```python
from build123d import *

# Parameters (mm, degrees)
F0_W      = 30
F0_H      = 30
F1_DEPTH  = 7
F3_DEPTH  = 7
F3_FACE_W = 4
F3_FACE_H = 7
F4_DEPTH  = 8


with BuildPart() as f1:
    # F0 (on Top) → F1 (new body)
    with BuildSketch(Plane.XY):
        Rectangle(F0_W, F0_H)
    extrude(amount=F1_DEPTH)

    # F2 (on face) → F3 (join)
    with BuildSketch(Plane.XY.offset(7)):
        with BuildLine():
            ThreePointArc((4, 0), (0, -4), (-4, 0))
            Line((-4, 0), (-8, 0))
            ThreePointArc((-8, 0), (0, -8), (8, 0))
            Line((8, 0), (4, 0))
        make_face()
    extrude(amount=F3_DEPTH)

    # F3_face (on face) → F4 (join)
    with BuildSketch(Plane(origin=(-6, 0, 10.5), x_dir=(-1, 0, 0), z_dir=(0, 1, 0))):
        Rectangle(F3_FACE_W, F3_FACE_H)
        with Locations((-12, 0)):
            Rectangle(F3_FACE_W, F3_FACE_H)
    extrude(amount=F4_DEPTH)


solid = f1.part
```
Work out the finished part from the listing and answer in its coordinate system (mm). A direction names the side the tool comes from. Give positions to 0.01 mm unless a question says otherwise; leave off trailing zeros. Loops run counter-clockwise (first coordinate to the right, second up) from the corner with the lowest first, then second, coordinate; pieces in that order, holes last. Notation, with made-up numbers: M -6.75,-6 L 39.25,-6 A15 cw 39.25,-1 Z; hole C -13,44.5 d2. An arc over 180 degrees is marked long. One line per item, written item: value. Start each with the question number.
1. Find section A-A (x = 0). Give the vertices of the cut face in (y, z).
2. Find section C-C (z = 11.5). Give the vertices of the cut face in (x, y), and give its area (3 significant figures).
3. Find section D-D (x = -9). Give the vertices of the cut face in (y, z), and give its area (3 significant figures).
4. Find section B-B (y = 7). Give the vertices of the cut face in (x, z).
5. Determine the mould class of faces 5 (the face through (-15, 0, 3)), 6 (the face through (0, 0, 0)), 7 (the face through (15, 0, 3)), 8 (the face through (0, 0, 7)) for opening direction X: released by +X, released by -X, zero draft, split by the parting line, or undercut.
6. Find the intervals of material crossed by probe 1 along X at (y, z) = (3, 12); probe 2 along Z at (x, y) = (3.5, 1); probe 3 along Y at (x, z) = (0, 9.25), in increasing order.
7. Which of the six approach directions +Z, -Z, +X, -X, +Y, -Y give full straight-line access (tool end or side, diameter ignored) to faces 1 (the face through (0, -8, 10)), 2 (the face through (-8, 4, 10)), 3 (the face through (4, 4, 10)), 4 (the face through (6, 8, 11))?
8. Each of these flat-tipped pins is pushed along its axis until it touches: P1, Ø3.5, axis at y = 2, z = 12, coming from the -X side; P2, Ø1.2, axis at x = -6, z = 10.5, coming from the +Y side; P3, Ø2, axis at y = 2.5, z = 10, coming from the +X side. Where does it stop, or does it pass through?
Reported:
1. outline: M -15,0 L 15,0 L 15,7 L -4,7 L -4,14 L -8,14 L -8,7 L -15,7 Z
2. outline: M -8,0 A8 ccw 8,0 L 8,8 L 4,8 L 4,0 A4 cw -4,0 L -4,8 L -8,8 Z
2. area: 139 mm²
3. outline: M -15,0 L 15,0 L 15,7 L -15,7 Z
3. area: 210 mm²
4. outline: M -15,0 L 15,0 L 15,7 L 8,7 L 8,14 L 4,14 L 4,7 L -4,7 L -4,14 L -8,14 L -8,7 L -15,7 Z
5. face 5: released by -X
5. face 6: zero draft
5. face 7: released by +X
5. face 8: undercut
6. probe 1: x = -8 to -4, 4 to 8
6. probe 2: z = 0 to 7
6. probe 3: y = -8 to -4
7. face 1: +Z, -Y
7. face 2: +Z, -X, +Y, -Y
7. face 3: +Z, +Y
7. face 4: +Z, +X, -X, +Y
8. P1: stops at x = -8
8. P2: stops at y = 8
8. P3: stops at x = 8
